from build123d import *

# Parameters (mm, degrees)
SKETCH1_R           = 3.6
BOSS_EXTRUDE1_DEPTH = 10
SKETCH2_R           = 8
BOSS_EXTRUDE2_DEPTH = 10
SKETCH3_R           = 3.25
CUT_EXTRUDE1_DEPTH  = 8
BOSS_EXTRUDE3_START = 10
SKETCH4_R           = 3.6
BOSS_EXTRUDE3_DEPTH = 10
FILLET1_R           = 2


with BuildPart() as part:
    # Sketch1 → Boss-Extrude1 (new body)
    with BuildSketch(Plane(origin=(0, 0, 0), x_dir=(1, 0, 0), z_dir=(0, 1, 0))):
        with Locations(Location((0, 0, 0), (0, 0, 270))):
            Circle(SKETCH1_R)
    extrude(amount=BOSS_EXTRUDE1_DEPTH)

    # Sketch2 → Boss-Extrude2 (add)
    with BuildSketch(Plane(origin=(0, 10, 0), x_dir=(1, 0, 0), z_dir=(0, 1, 0))):
        with Locations(Location((0, 0, 0), (0, 0, 270))):
            Circle(SKETCH2_R)
    extrude(amount=BOSS_EXTRUDE2_DEPTH)

    # Sketch3 → Cut-Extrude1 (cut)
    with BuildSketch(Plane(origin=(0, 20, 0), x_dir=(1, 0, 0), z_dir=(0, 1, 0))):
        with Locations(Location((0, 0, 0), (0, 0, 270))):
            Circle(SKETCH3_R)
    extrude(amount=-CUT_EXTRUDE1_DEPTH, mode=Mode.SUBTRACT)

    # Sketch4 → Boss-Extrude3 (add)
    with BuildSketch(Plane.XZ.offset(BOSS_EXTRUDE3_START)):
        with Locations(Location((0, 0, 0), (0, 0, 270))):
            Circle(SKETCH4_R)
    extrude(amount=-BOSS_EXTRUDE3_DEPTH)

    # Fillet1
    fillet1_edges = [part.edges().sort_by_distance(p)[0] for p in [
        (0, 10, -3.6),
    ]]
    fillet(fillet1_edges, radius=FILLET1_R)


solid = part.part
Can you work these out from the model? Positions are in its coordinate system, mm. A direction names the side the tool comes from. Coordinates: 2 decimals unless noted, no trailing zeros. Order: outer loops, then holes, each group sorted by start corner. A loop starts at its lowest first (then second) coordinate and runs counter-clockwise, first axis right, second up. Notation, with made-up numbers: (47.5, 69.25) -> (105.5, 69.25) arc R16 ccw to (105.5, 96.25) -> close; hole circle Ø8 at (8, 15). An arc over 180 degrees is marked (long way). Use one line per item in the form item = value.
Q1. Imagine slicing it at A-A, the plane z = 0. List the corners of the cut face in (x, y) for me, then the cut area to 3 significant figures.
From the geometry:
outline = (-8, 10) -> (-5.6, 10) arc R2 cw to (-3.6, 8) -> (-3.6, -10) -> (3.6, -10) -> (3.6, 8) arc R2 cw to (5.6, 10) -> (8, 10) -> (8, 20) -> (3.25, 20) -> (3.25, 12) -> (-3.25, 12) -> (-3.25, 20) -> (-8, 20) -> close
area = 254 mm²
Q2. Imagine slicing it at C-C, the plane y = 3.5. List the corners of the cut face in (x, z) for me, then the cut area to 3 significant figures.
From the geometry:
outline = circle Ø7.2 at (0, 0)
area = 40.7 mm²
Q3. Imagine slicing it at B-B, the plane x = 0. List the corners of the cut face in (y, z) for me.
From the geometry:
outline = (-10, -3.6) -> (8, -3.6) arc R2 cw to (10, -5.6) -> (10, -8) -> (20, -8) -> (20, -3.25) -> (12, -3.25) -> (12, 3.25) -> (20, 3.25) -> (20, 8) -> (10, 8) -> (10, 5.6) arc R2 cw to (8, 3.6) -> (-10, 3.6) -> close
Q4. I need wall thicknesses on L1, parallel to X at y = 15.5, z = 0; L2, parallel to Y at x = -5.5, z = -4.25; L3, parallel to Y at x = 1.5, z = 2. Which ranges of each line are inside material? Lowest first, please.
From the geometry:
L1 = -8 to -3.25, 3.25 to 8
L2 = 10 to 20
L3 = -10 to 12
Q5. We'd pull the mould along Z, two halves only. Please class faces 1 (the face through (-7.81, 14.93, -1.73)), 2 (the face through (0.1, 20, 3.4)), 3 (the face through (-1.978, 16.056, -2.579)), 4 (the face through (0, 12, 0)): released by +Z, released by -Z, zero draft, split by the parting line, or undercut.
From the geometry:
face_1 = split by the parting line
face_2 = zero draft
face_3 = undercut
face_4 = undercut
Q6. Imagine slicing it at D-D, the plane y = 15. List the corners of the cut face in (x, z) for me, then the cut area to 3 significant figures.
From the geometry:
outline = circle Ø16 at (0, 0); hole circle Ø6.5 at (0, 0)
area = 168 mm²
Q7. Which directions (+Z, -Z, +X, -X, +Y, -Y) give clear straight access to the entire face, cutting with the end or side of a thin tool? Please do faces 5 (the face through (5.45, 10, -1.89)), 6 (the face through (0, -10, 0)).
From the geometry:
face_5 = -Y
face_6 = +Z, -Z, +X, -X, -Y
Q8. Will these pins go through, and if not, where does the flat tip stop? P1, Ø1, axis at x = 6, y = 5, coming from the -Z side (1 decimal); P2, Ø4, axis at y = 2, z = -4.5, coming from the -X side; P3, Ø1, axis at x = -2.5, z = -6, coming from the -Y side.
From the geometry:
P1 = through
P2 = -2.59
P3 = 10
